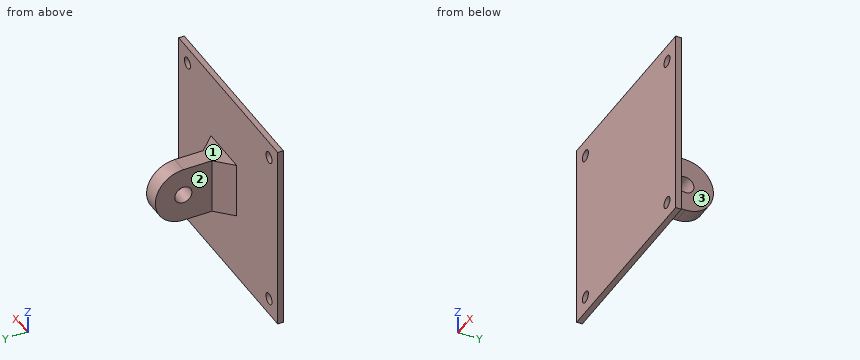
from build123d import *

# Parameters (mm, degrees)
SKETCH1_W           = 34
SKETCH1_H           = 34
SKETCH1_R           = 1.025
BOSS_EXTRUDE1_DEPTH = 1
SKETCH4_R           = 1.525
BOSS_EXTRUDE2_DEPTH = 3
CHAMFER1_SIZE       = 2.9


with BuildPart() as part:
    # Sketch1 → Boss-Extrude1 (new body)
    with BuildSketch(Plane(origin=(0, 0, 0), x_dir=(1, 0, 0), z_dir=(0, 1, 0))):
        Rectangle(SKETCH1_W, SKETCH1_H)
        with Locations(Location((-14, 14, 0), (0, 0, 270))):
            Circle(SKETCH1_R, mode=Mode.SUBTRACT)
        with Locations(Location((14, 14, 0), (0, 0, 270))):
            Circle(SKETCH1_R, mode=Mode.SUBTRACT)
        with Locations(Location((14, -14, 0), (0, 0, 270))):
            Circle(SKETCH1_R, mode=Mode.SUBTRACT)
        with Locations(Location((-14, -14, 0), (0, 0, 270))):
            Circle(SKETCH1_R, mode=Mode.SUBTRACT)
    extrude(amount=BOSS_EXTRUDE1_DEPTH)

    # Sketch4 → Boss-Extrude2 (add)
    with BuildSketch(Plane(origin=(0, 0, 0), x_dir=(0, 0, -1), z_dir=(1, 0, 0))):
        with BuildLine():
            Line((-5, 1), (5, 1))
            Line((5, 1), (5, 9))
            ThreePointArc((5, 9), (0, 14), (-5, 9))
            Line((-5, 9), (-5, 1))
        make_face()
        with Locations((0, 9)):
            Circle(SKETCH4_R, mode=Mode.SUBTRACT)
    extrude(amount=BOSS_EXTRUDE2_DEPTH)

    # Chamfer1
    chamfer1_edges = [part.edges().sort_by_distance(p)[0] for p in [
        (3, 1, 0),
        (0, 1, 0),
    ]]
    chamfer(chamfer1_edges, length=CHAMFER1_SIZE)


solid = part.part
Part model, mm, in its own coordinate system. Face numbers are marked on the shaded views. Give positions to 0.01 mm unless a question says otherwise; leave off trailing zeros. Order: outer loops, then holes, each group sorted by start corner. A loop starts at its lowest first (then second) coordinate and runs counter-clockwise, first axis right, second up. Notation, with made-up numbers: (-28, -13.75) -> (-24, -13.75) arc R22 cw to (-24, 6.25) -> close; hole circle Ø9 at (59.25, 2.25). An arc over 180 degrees is marked (long way). Use one line per item in the form item = value.
(1) Saw through at C-C (x = 14). Write the cut outline in (y, z) (3 decimals).
Solution:
outline = (0, -17) -> (1, -17) -> (1, -15.025) -> (0, -15.025) -> close; (0, -12.975) -> (1, -12.975) -> (1, 12.975) -> (0, 12.975) -> close; (0, 15.025) -> (1, 15.025) -> (1, 17) -> (0, 17) -> close
(2) Pull direction X, two halves, no side cores. Call the marked faces 1, 2 and 3: +X half, -X half, draft (parallel to the pull), parting line (faces both ways), or undercut.
Solution:
face_1 = draft
face_2 = -X half
face_3 = +X half
(3) Saw through at A-A (z = 0). Write the cut outline in (x, y) (3 decimals), then the cut area to 3 significant figures.
Solution:
outline = (-17, 0) -> (17, 0) -> (17, 1) -> (5.9, 1) -> (3, 3.9) -> (3, 7.475) -> (0, 7.475) -> (0, 3.9) -> (-2.9, 1) -> (-17, 1) -> close; (0, 10.525) -> (3, 10.525) -> (3, 14) -> (0, 14) -> close
area = 72.3 mm²
(4) Saw through at D-D (y = 8). Write the cut outline in (x, z).
Solution:
outline = (0, -5) -> (3, -5) -> (3, -1.15) -> (0, -1.15) -> close; (0, 1.15) -> (3, 1.15) -> (3, 5) -> (0, 5) -> close
(5) Drill centre lines: line 1 (X direction, y = 0.75, z = -14) (3 decimals); line 2 (Y direction, x = 1, z = 0) (3 decimals); line 3 (Y direction, x = -1, z = -9). Where is each one in solid material? Low to high. Write a range as from..to.
Solution:
line_1 = -17..-15.025, -12.975..12.975, 15.025..17
line_2 = 0..7.475, 10.525..14
line_3 = 0..1
(6) Flat gauge pins, fed straight in: P1, Ø6, axis at y = 10.5, z = 5, coming from the +X side; P2, Ø8, axis at y = 8, z = -2, coming from the -X side; P3, Ø3, axis at x = 9.5, z = 7, coming from the +Y side. Where does each tip first touch, or does it go through?
Solution:
P1 = 3
P2 = 0
P3 = 1
(7) Saw through at B-B (z = 14). Write the cut outline in (x, y) (3 decimals), then the cut area to 3 significant figures.
Solution:
outline = (-17, 0) -> (-15.025, 0) -> (-15.025, 1) -> (-17, 1) -> close; (-12.975, 0) -> (12.975, 0) -> (12.975, 1) -> (-12.975, 1) -> close; (15.025, 0) -> (17, 0) -> (17, 1) -> (15.025, 1) -> close
area = 29.9 mm²
